Geometry check sheet. Reference: the model listing, model coordinates, mm. A direction names the side the tool comes from. Give positions to 0.01 mm unless a question says otherwise; leave off trailing zeros. Write each loop counter-clockwise with the first axis right and the second up, starting at its lowest first coordinate (ties: lowest second). Pieces come first, ordered by that corner, then holes. Notation, with made-up numbers: (55, 16.5) -> (106, 16.5) arc R29 ccw to (106, 45.5) -> close; hole circle Ø5 at (7, -3.75). An arc over 180 degrees is marked (long way). Write item = value, one per line. Start each with the question number.
1. Cross-section at B-B, the plane x = -15.5. Record the cut outline in (y, z), plus the area to 3 significant figures.
2. Depth check by flat-ended pin: P1, Ø1.5, axis at y = 0.5, z = -0.5, coming from the -X side; P2, Ø4.5, axis at x = -25, y = 10, coming from the +Z side; P3, Ø12, axis at y = 0.5, z = -2.5, coming from the +X side; P4, Ø6, axis at x = -8.5, z = 52, coming from the -Y side. Enter the tip coordinate at first touch or a pass-through.
3. Cross-section at C-C, the plane z = -4. Record the cut outline in (x, y).
4. Thickness scan on line 1 along Y through (x, z) = (-46.5, 54); line 2 along Z through (x, y) = (-34.5, 9); line 3 along Y through (x, z) = (-48.5, 27). Record the ranges inside material, lowest first.
5. Cross-section at A-A, the plane y = 16.25. Record the cut outline in (x, z), plus the area to 3 significant figures.
6. Cross-section at D-D, the plane x = -47. Record the cut outline in (y, z), plus the area to 3 significant figures.
7. Set-up check for faces 1 (the flat face through (-39.613, 12, 40)), 2 (the flat face through (-9.613, 12, 40)), 3 (the flat face through (-25, 12, 36.689)): record each of +Z, -Z, +X, -X, +Y, -Y from which the full face is reachable in a straight line by a thin tool's end or side.
```python
from build123d import *

# Parameters (mm, degrees)
F0_R     = 30.807139
F1_DEPTH = 5
F2_R     = 40.117073
F3_DEPTH = 5
F4_W     = 30
F4_H     = 5.740043
F5_DEPTH = 20


with BuildPart() as f1:
    # F0 (on Front) → F1 (new body)
    with BuildSketch(Plane.XZ):
        with Locations((-24.092231, 22.158904)):
            Circle(F0_R)
    extrude(amount=F1_DEPTH)

    # F2 (on Front) → F3 (join)
    with BuildSketch(Plane.XZ):
        with Locations((-24.265252, 22.470835)):
            Circle(F2_R)
    extrude(amount=-F3_DEPTH)

    # F4 (on Front) → F5 (join)
    with BuildSketch(Plane.XZ):
        with Locations((-24.613258, 39.558847)):
            Rectangle(F4_W, F4_H)
    extrude(amount=-F5_DEPTH)


solid = f1.part
```
Answers:
q1.outline = (-5, -7.43) -> (0, -7.43) -> (0, -16.68) -> (5, -16.68) -> (5, 36.69) -> (20, 36.69) -> (20, 42.43) -> (5, 42.43) -> (5, 61.62) -> (0, 61.62) -> (0, 51.74) -> (-5, 51.74) -> close
q1.area = 773 mm^2
q2.P1 = -57.67
q2.P2 = 42.43
q2.P3 = 11.08
q2.P4 = -5
q3.outline = (-54.41, 0) -> (-40.36, 0) -> (-40.36, -5) -> (-7.82, -5) -> (-7.82, 0) -> (5.88, 0) -> (5.88, 5) -> (-54.41, 5) -> close
q4.line_1 = 0 to 5
q4.line_2 = 36.69 to 42.43
q4.line_3 = -5 to 5
q5.outline = (-39.61, 36.69) -> (-9.61, 36.69) -> (-9.61, 42.43) -> (-39.61, 42.43) -> close
q5.area = 172 mm^2
q6.outline = (-5, 1.56) -> (0, 1.56) -> (0, -10.58) -> (5, -10.58) -> (5, 55.52) -> (0, 55.52) -> (0, 42.76) -> (-5, 42.76) -> close
q6.area = 537 mm^2
q7.face_1 = +Z, -Z, -X, +Y
q7.face_2 = +Z, -Z, +X, +Y
q7.face_3 = -Z, +X, -X, +Y
